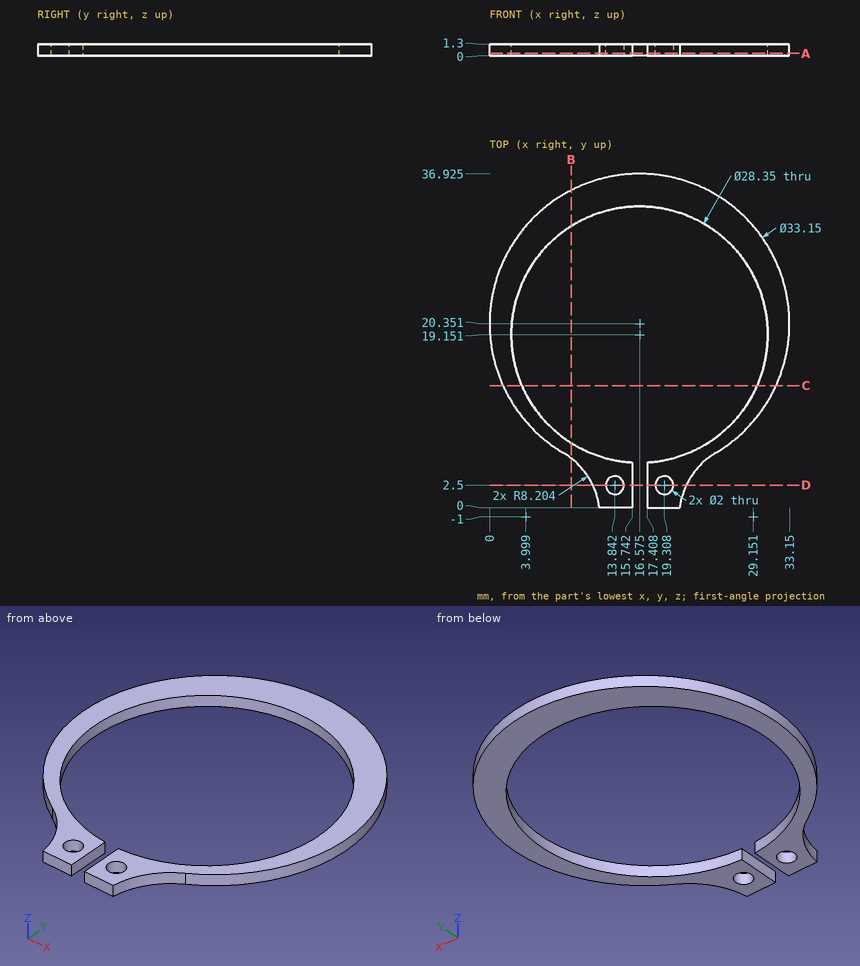
Geometry check sheet. Reference: drawing and pictorial views, mm from the part's lowest x, y, z. Round coordinates to 2 decimals unless told otherwise and drop trailing zeros. Order: outer loops, then holes, each group sorted by start corner. A loop starts at its lowest first (then second) coordinate and runs counter-clockwise, first axis right, second up. Notation, with made-up numbers: M 23,-22 L 78,-22 A12 ccw 78,-5 Z; hole C 53,53.25 d4. An arc over 180 degrees is marked long. Answer in a Markdown table with one row per item.
(1) Sectioned sample at A-A, the plane z = 0.25. State how many separate pieces and enclosed holes the cut face has, and give its area (3 significant figures).
Responses:
| item | result |
|---|---|
| separate pieces | 1 |
| enclosed holes | 2 |
| area | 261 mm² |
(2) Go/stop test with a flat-tipped pin: P1, Ø12, axis at x = 15.5, y = 24.5, coming from the -Z side. Record where the tip stops, or that it passes through.
Responses:
| item | result |
|---|---|
| P1 | passes through |
(3) Sectioned sample at D-D, the plane y = 2.5. Record the cut outline in (x, z).
Responses:
| item | result |
|---|---|
| outline | M 11.42,0 L 12.84,0 L 12.84,1.3 L 11.42,1.3 Z; M 14.84,0 L 15.74,0 L 15.74,1.3 L 14.84,1.3 Z; M 17.41,0 L 18.31,0 L 18.31,1.3 L 17.41,1.3 Z; M 20.31,0 L 21.73,0 L 21.73,1.3 L 20.31,1.3 Z |
(4) Sectioned sample at C-C, the plane y = 13.5. Record the cut outline in (x, z) (1 decimal).
Responses:
| item | result |
|---|---|
| outline | M 1.5,0 L 3.6,0 L 3.6,1.3 L 1.5,1.3 Z; M 29.6,0 L 31.7,0 L 31.7,1.3 L 29.6,1.3 Z |
(5) Sectioned sample at B-B, the plane x = 9. Record the cut outline in (y, z).
Responses:
| item | result |
|---|---|
| outline | M 5.5,0 L 7.17,0 L 7.17,1.3 L 5.5,1.3 Z; M 31.13,0 L 35.09,0 L 35.09,1.3 L 31.13,1.3 Z |
(6) Scan lines: probe 1 along Y at (x, z) = (20, 1.2) (1 decimal); probe 2 along X at (y, z) = (2, 1.15) (1 decimal); probe 3 along Y at (x, z) = (14, 0.6) (1 decimal). Record each from-to range of solid material in increasing order. Write a range as from..to.
Responses:
| item | result |
|---|---|
| probe 1 | y = 0..1.8, 3.2..5.4, 32.9..36.6 |
| probe 2 | x = 11.6..13, 14.7..15.7, 17.4..18.4, 20.2..21.5 |
| probe 3 | y = 0..1.5, 3.5..5.2, 33.1..36.7 |
